from build123d import *

# Parameters (mm, degrees)
SKETCH1_R               = 45
BOSS_EXTRUDE1_DEPTH     = 22.5
SKETCH2_R               = 45.69
BOSS_EXTRUDE2_DEPTH     = 2
SKETCH4_R               = 40
SKETCH4_R_2             = 37.69
CUT_EXTRUDE1_DEPTH      = 30
CUT_EXTRUDE2_DEPTH      = 79.741045205
CUT_EXTRUDE2_DEPTH_BACK = 79.741045205
SKETCH5_R               = 30
CUT_EXTRUDE3_DEPTH      = 79.741045205


with BuildPart() as part:
    # Sketch1 → Boss-Extrude1 (new, symmetric)
    with BuildSketch(Plane.XY):
        with Locations(Location((0, 0, 0), (0, 0, 180))):
            Circle(SKETCH1_R)
    extrude(amount=BOSS_EXTRUDE1_DEPTH, both=True)

    # Sketch2 → Boss-Extrude2 (add)
    with BuildSketch(Plane.XY.offset(22.5)):
        Circle(SKETCH2_R)
    boss_extrude2 = extrude(amount=-BOSS_EXTRUDE2_DEPTH)

    # Mirror1: Boss-Extrude2 across plane
    add(boss_extrude2.mirror(Plane.XY))

    # Sketch4 → Cut-Extrude1 (cut)
    with BuildSketch(Plane.XY):
        Circle(SKETCH4_R)
        Circle(SKETCH4_R_2, mode=Mode.SUBTRACT)
    extrude(amount=CUT_EXTRUDE1_DEPTH, mode=Mode.SUBTRACT)

    # Sketch5 → Cut-Extrude2 (cut, two sides: drawn at the far end of the back side and taken through both)
    with BuildSketch(Plane.XY.offset(22.5).offset(-CUT_EXTRUDE2_DEPTH_BACK)):
        Circle(SKETCH5_R)
    extrude(amount=CUT_EXTRUDE2_DEPTH + CUT_EXTRUDE2_DEPTH_BACK, mode=Mode.SUBTRACT)

    # Sketch6 → Cut-Extrude3 (cut, through all)
    with BuildSketch(Plane.XY.offset(22.5)):
        with BuildLine():
            Line((9, 20.17408731), (9, 33.20180718))
            ThreePointArc((9, 33.20180718), (0, 34.4), (-9, 33.20180718))
            Line((-9, 33.20180718), (-9, 20.17408731))
            Line((-9, 20.17408731), (9, 20.17408731))
        make_face()
    extrude(amount=-CUT_EXTRUDE3_DEPTH, mode=Mode.SUBTRACT)


solid = part.part
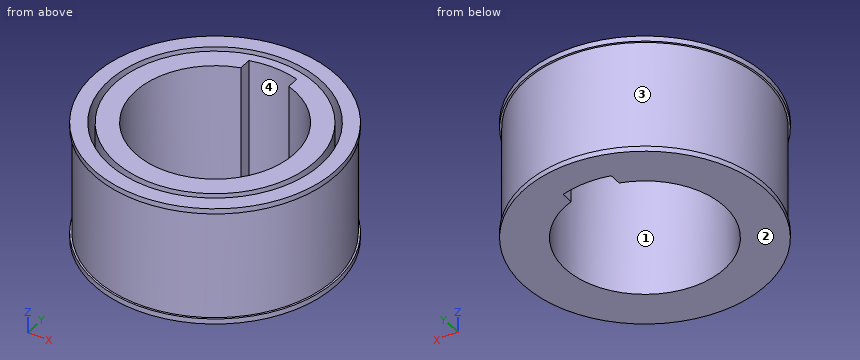
Verification items for the finished model (mm, model axes). Face numbers are marked on the shaded views. Round coordinates to 2 decimals unless told otherwise and drop trailing zeros. Loops run counter-clockwise (first coordinate to the right, second up) from the corner with the lowest first, then second, coordinate; pieces in that order, holes last. Notation, with made-up numbers: (18, 2.25) - (75, 2.25) arc R28 ccw to (75, 32.25) - close; hole circle Ø11 at (-17.75, 55.25). An arc over 180 degrees is marked (long way). Use one line per item in the form item = value.
1. Scan lines: probe 1 along Y at (x, z) = (0, 10); probe 2 along Y at (x, z) = (0, -12); probe 3 along Y at (x, z) = (8, 12). Record each from-to range of solid material in increasing order.
A:
probe_1 = -45 to -40, -37.69 to -30, 34.4 to 37.69, 40 to 45
probe_2 = -45 to -30, 34.4 to 45
probe_3 = -44.28 to -39.19, -36.83 to -28.91, 33.46 to 36.83, 39.19 to 44.28
2. Section check B-B on x = 0. Record the cut outline in (y, z), and give its area (3 significant figures).
A:
outline = (-45.69, -22.5) - (-30, -22.5) - (-30, 22.5) - (-37.69, 22.5) - (-37.69, 0) - (-40, 0) - (-40, 22.5) - (-45.69, 22.5) - (-45.69, 20.5) - (-45, 20.5) - (-45, -20.5) - (-45.69, -20.5) - close; (34.4, -22.5) - (45.69, -22.5) - (45.69, -20.5) - (45, -20.5) - (45, 20.5) - (45.69, 20.5) - (45.69, 22.5) - (40, 22.5) - (40, 0) - (37.69, 0) - (37.69, 22.5) - (34.4, 22.5) - close
area = 1,050 mm²
3. Draft check along Y on the marked faces 1, 2, 3 and 4. Enter one of: pulls with the +Y half, pulls with the -Y half, needs draft (parallel to the pull), parting line crosses it, or undercut.
A:
face_1 = undercut
face_2 = needs draft
face_3 = parting line crosses it
face_4 = undercut
4. Section check A-A on z = 6.5. Record the cut outline in (x, y), and give its area (3 significant figures).
A:
outline = circle Ø90 at (0, 0); circle Ø75.38 at (0, 0); hole circle Ø80 at (0, 0); hole (-9, 28.62) arc R30 ccw (long way) to (9, 28.62) - (9, 33.2) arc R34.4 ccw to (-9, 33.2) - close
area = 2,890 mm²
5. Section check C-C on y = 0. Record the cut outline in (x, z).
A:
outline = (-45.69, -22.5) - (-30, -22.5) - (-30, 22.5) - (-37.69, 22.5) - (-37.69, 0) - (-40, 0) - (-40, 22.5) - (-45.69, 22.5) - (-45.69, 20.5) - (-45, 20.5) - (-45, -20.5) - (-45.69, -20.5) - close; (30, -22.5) - (45.69, -22.5) - (45.69, -20.5) - (45, -20.5) - (45, 20.5) - (45.69, 20.5) - (45.69, 22.5) - (40, 22.5) - (40, 0) - (37.69, 0) - (37.69, 22.5) - (30, 22.5) - close
6. Section check D-D on z = -8.5. Record the cut outline in (x, y).
A:
outline = circle Ø90 at (0, 0); hole (-9, 28.62) arc R30 ccw (long way) to (9, 28.62) - (9, 33.2) arc R34.4 ccw to (-9, 33.2) - close
7. Gauge pin test, flat ends, axial feed: pin 1 Ø3 at (x, z) = (-1.5, -13) entering from +Y; pin 2 Ø3 at (y, z) = (22, 15.5) entering from -X; pin 3 Ø3.5 at (y, z) = (31.5, 1) entering from -X. Record the tip position at first contact, or that the pin passes through.
A:
pin_1 = 45
pin_2 = -40.06
pin_3 = -33.76
